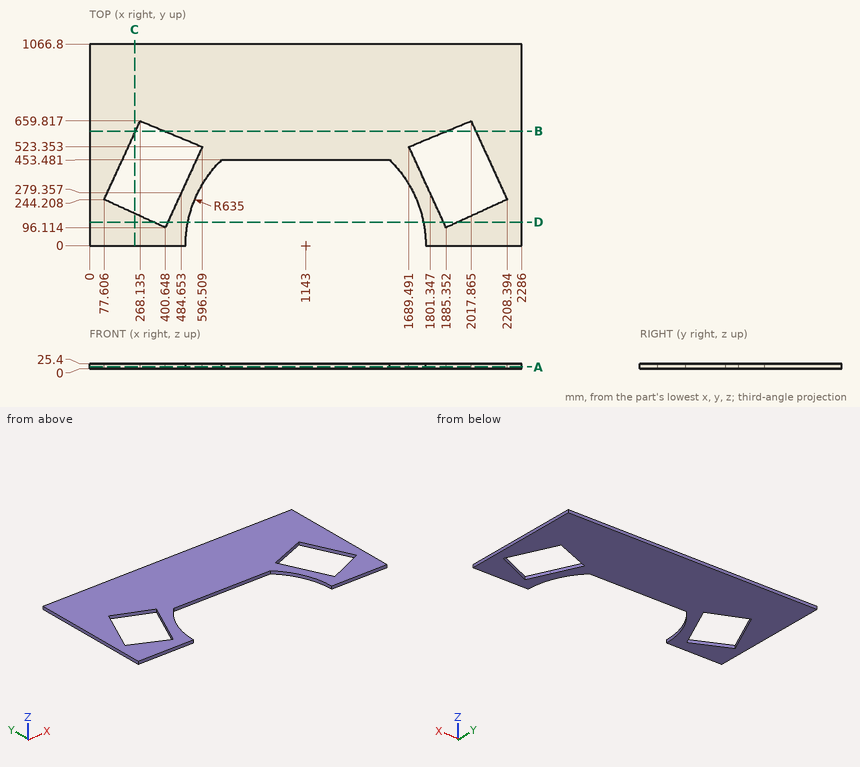
Could you check a few things on this drawing? It's one solid part, dimensions in mm from its lowest x, y, z. Coordinates: 2 decimals unless noted, no trailing zeros. Loops run counter-clockwise (first coordinate to the right, second up) from the corner with the lowest first, then second, coordinate; pieces in that order, holes last.
1. Imagine slicing it at C-C (x = 238). Please give me the cut outline in (y, z).
2. Imagine slicing it at A-A (z = 9.25). Please give me the cut outline in (x, y) (1 decimal).
3. I need wall thicknesses on L1, parallel to X at y = 593, z = 10.25 (1 decimal); L2, parallel to X at y = 188.5, z = 7.5 (1 decimal); L3, parallel to X at y = 495, z = 15. Which ranges of each line are inside material? Lowest first, please.
4. For P1, Ø8, axis at x = 1578.5, z = 9, coming from the -Y side, with a flat end and sliding along its axis, tell me the tip position at first contact or that it passes through.
5. Imagine slicing it at D-D (y = 125). Please give me the cut outline in (x, z) (1 decimal).
6. Imagine slicing it at B-B (y = 606.5). Please give me the cut outline in (x, z).
Computed values:
1. outline: (0, 0) - (170.68, 0) - (170.68, 25.4) - (0, 25.4) - close; (594.08, 0) - (1066.8, 0) - (1066.8, 25.4) - (594.08, 25.4) - close
2. outline: (0, 0) - (508, 0) arc R635 cw to (698.5, 453.5) - (1587.5, 453.5) arc R635 cw to (1778, 0) - (2286, 0) - (2286, 1066.8) - (0, 1066.8) - close; hole (77.6, 244.2) - (400.6, 96.1) - (596.5, 523.4) - (268.1, 659.8) - close; hole (1689.5, 523.4) - (1885.4, 96.1) - (2208.4, 244.2) - (2017.9, 659.8) - close
3. L1: x = 0 to 237.5, 428.9 to 1857.1, 2048.5 to 2286
3. L2: x = 0 to 199.1, 443 to 536.6, 1749.4 to 1843, 2086.9 to 2286
3. L3: x = 0 to 192.58, 583.51 to 1702.49, 2093.42 to 2286
4. P1: stops at y = 453.48
5. outline: (0, 0) - (337.6, 0) - (337.6, 25.4) - (0, 25.4) - close; (413.9, 0) - (520.4, 0) - (520.4, 25.4) - (413.9, 25.4) - close; (1765.6, 0) - (1872.1, 0) - (1872.1, 25.4) - (1765.6, 25.4) - close; (1948.4, 0) - (2286, 0) - (2286, 25.4) - (1948.4, 25.4) - close
6. outline: (0, 0) - (243.69, 0) - (243.69, 25.4) - (0, 25.4) - close; (396.43, 0) - (1889.57, 0) - (1889.57, 25.4) - (396.43, 25.4) - close; (2042.31, 0) - (2286, 0) - (2286, 25.4) - (2042.31, 25.4) - close
